Geometry check sheet. Reference: the model listing, model coordinates, mm. Give positions to 0.01 mm unless a question says otherwise; leave off trailing zeros. Write each loop counter-clockwise with the first axis right and the second up, starting at its lowest first coordinate (ties: lowest second). Pieces come first, ordered by that corner, then holes.
(1) Cross-section at B-B (y = 15.5). Record the boundary of the cut face in (x, z), and give its area (3 significant figures).
(2) Thickness scan on line 1 along Z through (x, y) = (1, 15.25); line 2 along Y through (x, z) = (0.35, -19.5). Record the ranges inside material, lowest first.
(3) Depth check by flat-ended pin: P1, Ø0.6, axis at x = 1, z = -22, coming from the -Y side. Enter the tip coordinate at first touch or a pass-through.
(4) Cross-section at A-A (x = 1.15). Record the boundary of the cut face in (y, z).
(5) Cross-section at C-C (z = -24). Record the boundary of the cut face in (x, y), and give its area (3 significant figures).
```python
from build123d import *

# Parameters (mm, degrees)
ESQUISSE1_W             = 50
ESQUISSE1_H             = 30
BOSS_EXTRU_1_DEPTH      = 2
ESQUISSE2_W             = 2
ESQUISSE2_H             = 15
ENL_V_MAT_EXTRU_1_DEPTH = 2
ESQUISSE3_W             = 15.005230118
ESQUISSE3_H             = 2
ENL_V_MAT_EXTRU_2_DEPTH = 2


with BuildPart() as part:
    # Esquisse1 → Boss.-Extru.1 (new body)
    with BuildSketch(Plane(origin=(0, 0, 0), x_dir=(0, 0, -1), z_dir=(1, 0, 0))):
        with Locations((25, 15)):
            Rectangle(ESQUISSE1_W, ESQUISSE1_H)
    extrude(amount=BOSS_EXTRU_1_DEPTH)

    # Esquisse2 → Enlèv. mat.-Extru.1 (cut)
    with BuildSketch(Plane(origin=(2, 0, 0), x_dir=(0, 0, -1), z_dir=(1, 0, 0))):
        with Locations((1, 15)):
            Rectangle(ESQUISSE2_W, ESQUISSE2_H)
        with Locations((49, 15)):
            Rectangle(ESQUISSE2_W, ESQUISSE2_H)
    extrude(amount=-ENL_V_MAT_EXTRU_1_DEPTH, mode=Mode.SUBTRACT)

    # Esquisse3 → Enlèv. mat.-Extru.2 (cut)
    with BuildSketch(Plane(origin=(2, 0, 0), x_dir=(0, 0, -1), z_dir=(1, 0, 0))):
        with Locations((25, 1)):
            Rectangle(ESQUISSE3_W, ESQUISSE3_H)
    extrude(amount=-ENL_V_MAT_EXTRU_2_DEPTH, mode=Mode.SUBTRACT)


solid = part.part
```
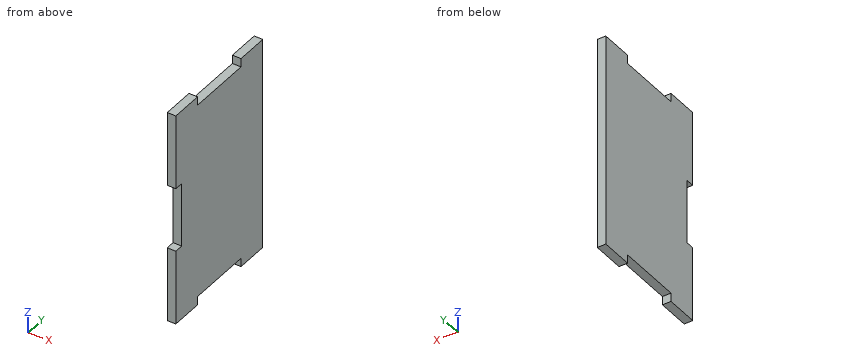
Reply:
1. outline: (0, -48) - (2, -48) - (2, -2) - (0, -2) - close
1. area: 92.0 mm2
2. line 1: z = -48 to -2
2. line 2: y = 2 to 30
3. P1: stops at y = 2
4. outline: (0, -50) - (7.5, -50) - (7.5, -48) - (22.5, -48) - (22.5, -50) - (30, -50) - (30, 0) - (22.5, 0) - (22.5, -2) - (7.5, -2) - (7.5, 0) - (0, 0) - (0, -17.5) - (2, -17.5) - (2, -32.5) - (0, -32.5) - close
5. outline: (0, 2) - (2, 2) - (2, 30) - (0, 30) - close
5. area: 56.0 mm2
